from build123d import *

# Parameters (mm, degrees)
SKETCH1_R           = 10
BOSS_EXTRUDE1_DEPTH = 40
SKETCH2_R           = 5
BOSS_EXTRUDE2_DEPTH = 25
CIRPATTERN1_COUNT   = 3


with BuildPart() as part:
    # Sketch1 → Boss-Extrude1 (new body)
    with BuildSketch(Plane(origin=(0, 0, 0), x_dir=(1, 0, 0), z_dir=(0, 1, 0))):
        with BuildLine():
            Line((-10, 114.641016151), (-20, 114.641016151))
            Line((-20, 114.641016151), (-20, 34.641016151))
            ThreePointArc((-20, 34.641016151), (-34.641016151, 20), (-40, 0))
            Line((-40, 0), (-109.282032303, -40))
            Line((-109.282032303, -40), (-104.282032303, -48.660254038))
            Line((-104.282032303, -48.660254038), (-69.641016151, -28.660254038))
            Line((-69.641016151, -28.660254038), (-59.641016151, -45.980762114))
            Line((-59.641016151, -45.980762114), (-94.282032303, -65.980762114))
            Line((-94.282032303, -65.980762114), (-89.282032303, -74.641016151))
            Line((-89.282032303, -74.641016151), (-20, -34.641016151))
            ThreePointArc((-20, -34.641016151), (0, -40), (20, -34.641016151))
            Line((20, -34.641016151), (89.282032303, -74.641016151))
            Line((89.282032303, -74.641016151), (94.282032303, -65.980762114))
            Line((94.282032303, -65.980762114), (59.641016151, -45.980762114))
            Line((59.641016151, -45.980762114), (69.641016151, -28.660254038))
            Line((69.641016151, -28.660254038), (104.282032303, -48.660254038))
            Line((104.282032303, -48.660254038), (109.282032303, -40))
            Line((109.282032303, -40), (40, 0))
            ThreePointArc((40, 0), (34.641016151, 20), (20, 34.641016151))
            Line((20, 34.641016151), (20, 114.641016151))
            Line((20, 114.641016151), (10, 114.641016151))
            Line((10, 114.641016151), (10, 74.641016151))
            Line((10, 74.641016151), (-10, 74.641016151))
            Line((-10, 74.641016151), (-10, 114.641016151))
        make_face()
        with Locations(Location((0, 0, 0), (0, 0, 270))):
            Circle(SKETCH1_R, mode=Mode.SUBTRACT)
    extrude(amount=BOSS_EXTRUDE1_DEPTH)

    # Sketch2 → Boss-Extrude2 (add)
    with BuildSketch(Plane(origin=(-10, 0, 0), x_dir=(0, 0, -1), z_dir=(1, 0, 0))):
        with Locations((99.641016151, 20)):
            Circle(SKETCH2_R)
    boss_extrude2 = extrude(amount=BOSS_EXTRUDE2_DEPTH)

    # CirPattern1: Boss-Extrude2 ×3 about axis
    cirpattern1_axis = Axis((0, 40, 0), (0, 1, 0))
    for i in range(1, CIRPATTERN1_COUNT):
        add(boss_extrude2.rotate(cirpattern1_axis, i * 360 / CIRPATTERN1_COUNT))


solid = part.part
Geometry: final body of the model. Coordinates: model frame, mm. A direction names the side the tool comes from. Give positions to 0.01 mm unless a question says otherwise; leave off trailing zeros. Loops run counter-clockwise (first coordinate to the right, second up) from the corner with the lowest first, then second, coordinate; pieces in that order, holes last. Notation, with made-up numbers: (37, 38.5) - (81, 38.5) arc R6 cw to (81, 44.5) - close; hole circle Ø2 at (-17, -25.5). An arc over 180 degrees is marked (long way). One line per question, with ' | ' between items. Start each with the question number.
(1) Section query A-A on x = 0. Return loops of the section in (y, z).
(2) Section query B-B on y = 34. Return loops of the section in (x, z), then the cut area to 3 significant figures.
(3) Reachability of faces 1 (the flat face through (73.36, 19.72, 53.9)), 2 (the flat face through (20, 20, -74)), 3 (the flat face through (-55.126, 19.72, 54.921)), 4 (the flat face through (0, 20, -74.641)) from +Z, -Z, +X, -X, +Y, -Y: full face, straight path, thin tool, end or side. Return the list, or none.
(4) Section query D-D on z = 55. Count the separate pieces of the cut face and the enclosed holes in it, then the cut area to 3 significant figures.
(5) Contact query for flat-ended pins moving along their axis: pin 1 (8 mm diameter, centred on x = -57, y = 11.5, fed in from +Z); pin 2 (20 mm diameter, centred on y = 12, z = -85.5, fed in from -X); pin 3 (6 mm diameter, centred on x = -6.5, z = -75.5, fed in from -Y); pin 4 (1 mm diameter, centred on y = 27.5, z = -3, fed in from -X). Output: stop coordinate, or through.
(6) Section query C-C on z = -39.5. Return loops of the section in (x, y), then the cut area to 3 significant figures.
(7) Ray query, line 1 (X direction, y = 30, z = -98); line 2 (X direction, y = 20, z = 0); line 3 (Z direction, x = 3.5, y = 19). Return the intervals inside material, ascending. Write a range as from..to.
(8) Pull-direction query (X, two-part tool) for faces 5 (the cylindrical face through (34.787, 19.72, -19.746)), 6 (the flat face through (-74.16, 19.72, 19.72)), 7 (the flat face through (15, 20, -114.641)), 8 (the cylindrical face through (-88.22, 15.564, 51.095)); classes: released by +X, released by -X, zero draft, split by the parting line, or undercut.
The answers:
1) outline: (0, -74.64) - (40, -74.64) - (40, -10) - (0, -10) - close; (0, 10) - (40, 10) - (40, 40) - (0, 40) - close; circle Ø10 at (20, -99.64)
2) outline: (-109.28, 40) - (-40, 0) arc R40 ccw to (-20, -34.64) - (-20, -114.64) - (-10, -114.64) - (-10, -74.64) - (10, -74.64) - (10, -114.64) - (20, -114.64) - (20, -34.64) arc R40 ccw to (40, 0) - (109.28, 40) - (104.28, 48.66) - (69.64, 28.66) - (59.64, 45.98) - (94.28, 65.98) - (89.28, 74.64) - (20, 34.64) arc R40 ccw to (-20, 34.64) - (-89.28, 74.64) - (-94.28, 65.98) - (-59.64, 45.98) - (-69.64, 28.66) - (-104.28, 48.66) - close; hole circle Ø20 at (0, 0) | area: 11,500 mm2
3) face 1: none | face 2: -Z, +X, +Y, -Y | face 3: +Z, +Y, -Y | face 4: +Y, -Y
4) separate pieces: 4 | enclosed holes: 0 | area: 1,780 mm2
5) pin 1: z = 58.31 | pin 2: x = -20 | pin 3: y = 0 | pin 4: x = -39.92
6) outline: (-20, 0) - (20, 0) - (20, 40) - (-20, 40) - close | area: 1,600 mm2
7) line 1: -20..-10, 10..20 | line 2: -40..-10, 10..40 | line 3: -104.54..-94.74, -74.64..-9.37, 9.37..39.85
8) face 5: released by +X | face 6: released by -X | face 7: zero draft | face 8: undercut
